```python
from build123d import *

# Parameters (mm, degrees)
F0_R     = 14.224
F1_DEPTH = 50.8
F2_W     = 19.05
F2_H     = 19.05
F3_DEPTH = 10.16
F4_R     = 4.7625
F5_DEPTH = 25.4
F6_R     = 9.52499


# Not quite as in the source:
# - a fillet or chamfer is up to 0.001 mm smaller than in the source, because OpenCascade refuses the exact size


with BuildPart() as f1:
    # F0 (on Front) → F1 (new body)
    with BuildSketch(Plane.XZ):
        Circle(F0_R)
    extrude(amount=F1_DEPTH)

    # F2 (on Right) → F3 (join, symmetric)
    with BuildSketch(Plane.YZ):
        with Locations((9.525, 0)):
            Rectangle(F2_W, F2_H)
    extrude(amount=F3_DEPTH, both=True)

    # F4 (on face) → F5 (cut)
    with BuildSketch(Plane.YZ.offset(10.16)):
        with Locations((9.525, 0)):
            Circle(F4_R)
    extrude(amount=-F5_DEPTH, mode=Mode.SUBTRACT)

    # F6 (radius 9.525 in the source; OpenCascade refuses exactly that, so slightly less here)
    f6_edges = [f1.edges().sort_by_distance(p)[0] for p in [
        (0, 19.05, 9.525),
        (0, 19.05, -9.525),
    ]]
    fillet(f6_edges, radius=F6_R)


solid = f1.part
```
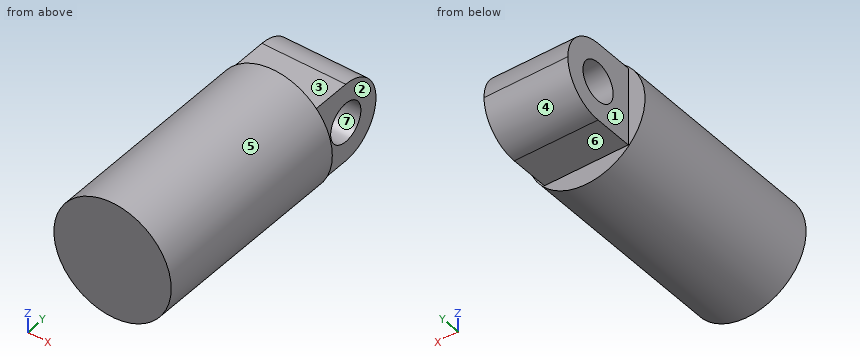
Build history of the part. All positions in model axes, mm. Face numbers are marked on the shaded views. A direction names the side the tool comes from. Give positions to 0.01 mm unless a question says otherwise; leave off trailing zeros. Order: outer loops, then holes, each group sorted by start corner. A loop starts at its lowest first (then second) coordinate and runs counter-clockwise, first axis right, second up. Notation, with made-up numbers: M -1.5,71.5 L 22.5,71.5 A29 ccw 22.5,109.5 Z; hole C 81,-23 d9. An arc over 180 degrees is marked long. Return JSON: item names as keys, results as strings.
Q1. Two-plate mould, pull along Z, no slides. Class the marked faces 5, 6 and 7: pulls with the +Z half, pulls with the -Z half, needs draft (parallel to the pull), parting line crosses it, or undercut.
Answer list:
{"face 5": "parting line crosses it", "face 6": "pulls with the -Z half", "face 7": "undercut"}
Q2. Wall check: probe 1 along X at (y, z) = (7, 9.25); probe 2 along Y at (x, z) = (9.5, 10); probe 3 along Z at (x, y) = (0, -46.5). Give the ranges that are in metal, low to high. Write a range as from..to.
Answer list:
{"probe 1": "x = -10.16..10.16", "probe 2": "y = -50.8..0", "probe 3": "z = -14.22..14.22"}
Q3. Flat gauge pins, fed straight in: pin 1 (8 mm diameter, centred on x = 3, y = 6, fed in from -Z) (3 decimals); pin 2 (1.5 mm diameter, centred on y = -38, z = 7, fed in from -X); pin 3 (10 mm diameter, centred on x = 11, y = -40.5, fed in from -Z); pin 4 (7.5 mm diameter, centred on y = 9.525, z = 0, fed in from -X). Where does each tip first touch, or does it go through?
Answer list:
{"pin 1": "stops at z = -9.525", "pin 2": "stops at x = -12.78", "pin 3": "stops at z = -12.9", "pin 4": "passes through"}
Q4. Band-saw the part on D-D (y = -12). Give the cut face in (x, z).
Answer list:
{"outline": "C 0,0 d28.45"}
Q5. Band-saw the part on A-A (y = 12). Give the cut face in (x, z), then the cut area to 3 significant figures.
Answer list:
{"outline": "M -10.16,-9.2 L 10.16,-9.2 L 10.16,-4.07 L -10.16,-4.07 Z; M -10.16,4.07 L 10.16,4.07 L 10.16,9.2 L -10.16,9.2 Z", "area": "208 mm^2"}
Q6. Band-saw the part on B-B (z = 2). Give the cut face in (x, y), then the cut area to 3 significant figures.
Answer list:
{"outline": "M -14.08,-50.8 L 14.08,-50.8 L 14.08,0 L 10.16,0 L 10.16,5.2 L -10.16,5.2 L -10.16,0 L -14.08,0 Z; M -10.16,13.85 L 10.16,13.85 L 10.16,18.84 L -10.16,18.84 Z", "area": "1,640 mm^2"}
Q7. 3-axis set-ups, long thin cutter, end or side, ignore diameter. For the marked faces 1, 2, 3 and 4: which of +Z, -Z, +X, -X, +Y, -Y reach the whole face in a straight line?
Answer list:
{"face 1": "+Z, -Z, -X, +Y", "face 2": "+Z, -Z, +X, +Y", "face 3": "+Z, +X, -X, +Y", "face 4": "-Z, +X, -X, +Y"}
